from build123d import *

# Parameters (mm, degrees)
SKETCH_1_W           = 300
SKETCH_1_H           = 100
EXTRUDE_1_DEPTH      = 16
SKETCH_2_W           = 30
SKETCH_2_H           = 30
CUT_EXTRUDE_1_DEPTH  = 8
SKETCH_3_R           = 12.5
CUT_EXTRUDE_2_DEPTH  = 14
CUT_EXTRUDE_3_REACH  = 318.632
SKETCH_4_W           = 50
SKETCH_4_H           = 35
SKETCH_7_W           = 35
SKETCH_7_H           = 16
EXTRUDE_2_DEPTH      = 20
SKETCH_8_W           = 35
SKETCH_8_H           = 16
EXTRUDE_3_DEPTH      = 20
SKETCH_9_W           = 20
SKETCH_9_H           = 10
EXTRUDE_4_DEPTH      = 25
FILLET_1_R           = 1
FILLET_2_R           = 1
SKETCH_13_W          = 35
SKETCH_13_H          = 16
EXTRUDE_6_DEPTH      = 4
SKETCH_14_W          = 35
SKETCH_14_H          = 16
EXTRUDE_7_DEPTH      = 4
SKETCH_17_W          = 35
SKETCH_17_H          = 16
EXTRUDE_8_DEPTH      = 1
SKETCH_18_W          = 35
SKETCH_18_H          = 16
EXTRUDE_9_DEPTH      = 1
SKETCH_19_R          = 2.25
CUT_EXTRUDE_8_DEPTH  = 5
CUT_EXTRUDE_START    = -5
SKETCH_20_R          = 2.25
CUT_EXTRUDE_9_DEPTH  = 5
SKETCH_21_R          = 1.45
CUT_EXTRUDE_10_DEPTH = 5
SKETCH_22_R          = 2.25
CUT_EXTRUDE_11_DEPTH = 5
SKETCH_23_R          = 1.45
CUT_EXTRUDE_12_DEPTH = 5
SKETCH_24_R          = 2.25
CUT_EXTRUDE_13_DEPTH = 5


with BuildPart() as part:
    # 草图1 → 凸台-拉伸1 (new body)
    with BuildSketch(Plane(origin=(0, 0, 0), x_dir=(1, 0, 0), z_dir=(0, 1, 0))):
        with Locations((-150, 50)):
            Rectangle(SKETCH_1_W, SKETCH_1_H)
    extrude(amount=EXTRUDE_1_DEPTH)

    # 草图2 → 切除-拉伸1 (cut)
    with BuildSketch(Plane(origin=(0, 16, 0), x_dir=(1, 0, 0), z_dir=(0, 1, 0))):
        with Locations((-150, 50)):
            Rectangle(SKETCH_2_W, SKETCH_2_H)
    extrude(amount=-CUT_EXTRUDE_1_DEPTH, mode=Mode.SUBTRACT)

    # 草图3 → 切除-拉伸2 (cut)
    with BuildSketch(Plane(origin=(0, 8, 0), x_dir=(1, 0, 0), z_dir=(0, 1, 0))):
        with Locations(Location((-150, 50, 0), (0, 0, 270))):
            Circle(SKETCH_3_R)
    extrude(amount=-CUT_EXTRUDE_2_DEPTH, mode=Mode.SUBTRACT)

    # 草图4 → 切除-拉伸3 (cut, up to next)
    with BuildSketch(Plane(origin=(0, 16, 0), x_dir=(1, 0, 0), z_dir=(0, 1, 0)), mode=Mode.PRIVATE) as cut_extrude_3_sk1:
        with Locations((-270, 72.5)):
            Rectangle(SKETCH_4_W, SKETCH_4_H)
    cut_extrude_3_tool1 = extrude(cut_extrude_3_sk1.sketch, amount=-CUT_EXTRUDE_3_REACH, mode=Mode.PRIVATE) & part.part
    # 草图4 → 切除-拉伸3 (cut, up to next)
    with BuildSketch(Plane(origin=(0, 16, 0), x_dir=(1, 0, 0), z_dir=(0, 1, 0)), mode=Mode.PRIVATE) as cut_extrude_3_sk2:
        with Locations((-270, 27.5)):
            Rectangle(SKETCH_4_W, SKETCH_4_H)
    cut_extrude_3_tool2 = extrude(cut_extrude_3_sk2.sketch, amount=-CUT_EXTRUDE_3_REACH, mode=Mode.PRIVATE) & part.part
    # 草图4 → 切除-拉伸3 (cut, up to next)
    with BuildSketch(Plane(origin=(0, 16, 0), x_dir=(1, 0, 0), z_dir=(0, 1, 0)), mode=Mode.PRIVATE) as cut_extrude_3_sk3:
        with Locations((-210, 72.5)):
            Rectangle(SKETCH_4_W, SKETCH_4_H)
    cut_extrude_3_tool3 = extrude(cut_extrude_3_sk3.sketch, amount=-CUT_EXTRUDE_3_REACH, mode=Mode.PRIVATE) & part.part
    # 草图4 → 切除-拉伸3 (cut, up to next)
    with BuildSketch(Plane(origin=(0, 16, 0), x_dir=(1, 0, 0), z_dir=(0, 1, 0)), mode=Mode.PRIVATE) as cut_extrude_3_sk4:
        with Locations((-210, 27.5)):
            Rectangle(SKETCH_4_W, SKETCH_4_H)
    cut_extrude_3_tool4 = extrude(cut_extrude_3_sk4.sketch, amount=-CUT_EXTRUDE_3_REACH, mode=Mode.PRIVATE) & part.part
    # 草图4 → 切除-拉伸3 (cut, up to next)
    with BuildSketch(Plane(origin=(0, 16, 0), x_dir=(1, 0, 0), z_dir=(0, 1, 0)), mode=Mode.PRIVATE) as cut_extrude_3_sk5:
        with Locations((-30, 27.5)):
            Rectangle(SKETCH_4_W, SKETCH_4_H)
    cut_extrude_3_tool5 = extrude(cut_extrude_3_sk5.sketch, amount=-CUT_EXTRUDE_3_REACH, mode=Mode.PRIVATE) & part.part
    # 草图4 → 切除-拉伸3 (cut, up to next)
    with BuildSketch(Plane(origin=(0, 16, 0), x_dir=(1, 0, 0), z_dir=(0, 1, 0)), mode=Mode.PRIVATE) as cut_extrude_3_sk6:
        with Locations((-90, 27.5)):
            Rectangle(SKETCH_4_W, SKETCH_4_H)
    cut_extrude_3_tool6 = extrude(cut_extrude_3_sk6.sketch, amount=-CUT_EXTRUDE_3_REACH, mode=Mode.PRIVATE) & part.part
    # 草图4 → 切除-拉伸3 (cut, up to next)
    with BuildSketch(Plane(origin=(0, 16, 0), x_dir=(1, 0, 0), z_dir=(0, 1, 0)), mode=Mode.PRIVATE) as cut_extrude_3_sk7:
        with Locations((-90, 72.5)):
            Rectangle(SKETCH_4_W, SKETCH_4_H)
    cut_extrude_3_tool7 = extrude(cut_extrude_3_sk7.sketch, amount=-CUT_EXTRUDE_3_REACH, mode=Mode.PRIVATE) & part.part
    # 草图4 → 切除-拉伸3 (cut, up to next)
    with BuildSketch(Plane(origin=(0, 16, 0), x_dir=(1, 0, 0), z_dir=(0, 1, 0)), mode=Mode.PRIVATE) as cut_extrude_3_sk8:
        with Locations((-30, 72.5)):
            Rectangle(SKETCH_4_W, SKETCH_4_H)
    cut_extrude_3_tool8 = extrude(cut_extrude_3_sk8.sketch, amount=-CUT_EXTRUDE_3_REACH, mode=Mode.PRIVATE) & part.part
    add(cut_extrude_3_tool1.solids().sort_by_distance((-270, 16, -72.5))[0], mode=Mode.SUBTRACT)
    add(cut_extrude_3_tool2.solids().sort_by_distance((-270, 16, -27.5))[0], mode=Mode.SUBTRACT)
    add(cut_extrude_3_tool3.solids().sort_by_distance((-210, 16, -72.5))[0], mode=Mode.SUBTRACT)
    add(cut_extrude_3_tool4.solids().sort_by_distance((-210, 16, -27.5))[0], mode=Mode.SUBTRACT)
    add(cut_extrude_3_tool5.solids().sort_by_distance((-30, 16, -27.5))[0], mode=Mode.SUBTRACT)
    add(cut_extrude_3_tool6.solids().sort_by_distance((-90, 16, -27.5))[0], mode=Mode.SUBTRACT)
    add(cut_extrude_3_tool7.solids().sort_by_distance((-90, 16, -72.5))[0], mode=Mode.SUBTRACT)
    add(cut_extrude_3_tool8.solids().sort_by_distance((-30, 16, -72.5))[0], mode=Mode.SUBTRACT)

    # 草图7 → 凸台-拉伸2 (add)
    with BuildSketch(Plane.ZY.offset(185)):
        with Locations((-27.5, 8)):
            Rectangle(SKETCH_7_W, SKETCH_7_H)
        with Locations((-72.5, 8)):
            Rectangle(SKETCH_7_W, SKETCH_7_H)
    extrude(amount=EXTRUDE_2_DEPTH)

    # 草图8 → 凸台-拉伸3 (add)
    with BuildSketch(Plane(origin=(-115, 0, 0), x_dir=(0, 0, -1), z_dir=(1, 0, 0))):
        with Locations((27.5, 8)):
            Rectangle(SKETCH_8_W, SKETCH_8_H)
        with Locations((72.5, 8)):
            Rectangle(SKETCH_8_W, SKETCH_8_H)
    extrude(amount=EXTRUDE_3_DEPTH)

    # 草图9 → 凸台-拉伸4 (add)
    with BuildSketch(Plane.XZ):
        with Locations((-250, -95)):
            Rectangle(SKETCH_9_W, SKETCH_9_H)
    extrude(amount=EXTRUDE_4_DEPTH)

    # 圆角1
    fillet_1_edges = [part.edges().sort_by_distance(p)[0] for p in [
        (-150, 8, -62.5),
    ]]
    fillet(fillet_1_edges, radius=FILLET_1_R)

    # 圆角2
    fillet_2_edges = [part.edges().sort_by_distance(p)[0] for p in [
        (-135, 16, -50),
        (-150, 16, -65),
        (-165, 16, -50),
        (-150, 16, -35),
    ]]
    fillet(fillet_2_edges, radius=FILLET_2_R)

    # 草图13 → 凸台-拉伸6 (add)
    with BuildSketch(Plane.ZY.offset(5)):
        with Locations((-72.5, 8)):
            Rectangle(SKETCH_13_W, SKETCH_13_H)
        with Locations((-27.5, 8)):
            Rectangle(SKETCH_13_W, SKETCH_13_H)
    extrude(amount=EXTRUDE_6_DEPTH)

    # 草图14 → 凸台-拉伸7 (add)
    with BuildSketch(Plane(origin=(-295, 0, 0), x_dir=(0, 0, -1), z_dir=(1, 0, 0))):
        with Locations((72.5, 8)):
            Rectangle(SKETCH_14_W, SKETCH_14_H)
        with Locations((27.5, 8)):
            Rectangle(SKETCH_14_W, SKETCH_14_H)
    extrude(amount=EXTRUDE_7_DEPTH)

    # 草图17 → 凸台-拉伸8 (add)
    with BuildSketch(Plane(origin=(-291, 0, 0), x_dir=(0, 0, -1), z_dir=(1, 0, 0))):
        with Locations((27.5, 8)):
            Rectangle(SKETCH_17_W, SKETCH_17_H)
        with Locations((72.5, 8)):
            Rectangle(SKETCH_17_W, SKETCH_17_H)
    extrude(amount=EXTRUDE_8_DEPTH)

    # 草图18 → 凸台-拉伸9 (add)
    with BuildSketch(Plane.ZY.offset(9)):
        with Locations((-27.5, 8)):
            Rectangle(SKETCH_18_W, SKETCH_18_H)
        with Locations((-72.5, 8)):
            Rectangle(SKETCH_18_W, SKETCH_18_H)
    extrude(amount=EXTRUDE_9_DEPTH)

    # 草图19 → 切除-拉伸8 (cut)
    with BuildSketch(Plane(origin=(0, 16, 0), x_dir=(1, 0, 0), z_dir=(0, 1, 0))):
        with Locations(Location((-295, 95, 0), (0, 0, 270))):
            Circle(SKETCH_19_R)
        with Locations(Location((-295, 5, 0), (0, 0, 90))):
            Circle(SKETCH_19_R)
        with Locations(Location((-5, 5, 0), (0, 0, 270))):
            Circle(SKETCH_19_R)
        with Locations(Location((-5, 95, 0), (0, 0, 90))):
            Circle(SKETCH_19_R)
    extrude(amount=-CUT_EXTRUDE_8_DEPTH, mode=Mode.SUBTRACT)

    # 草图20 → 切除-拉伸9 (cut)
    with BuildSketch(Plane.XZ.offset(CUT_EXTRUDE_START)):
        with Locations(Location((-295, -95, 0), (0, 0, 90))):
            Circle(SKETCH_20_R)
        with Locations(Location((-295, -5, 0), (0, 0, 270))):
            Circle(SKETCH_20_R)
        with Locations(Location((-5, -95, 0), (0, 0, 270))):
            Circle(SKETCH_20_R)
        with Locations(Location((-5, -5, 0), (0, 0, 90))):
            Circle(SKETCH_20_R)
    extrude(amount=CUT_EXTRUDE_9_DEPTH, mode=Mode.SUBTRACT)

    # 草图21 → 切除-拉伸10 (cut)
    with BuildSketch(Plane(origin=(-100.276222054, 16, -200.091791604), x_dir=(-0.00184091553368713, 0, -0.9999983055135633), z_dir=(0, 1, 0))):
        with Locations(Location((-104.543338614, 26.416278164, 0), (0, 0, 179.89452325))):
            Circle(SKETCH_21_R)
        with Locations(Location((-121.543309808, 26.447573728, 0), (0, 0, 179.89452325))):
            Circle(SKETCH_21_R)
        with Locations(Location((-121.456786778, 73.447494087, 0), (0, 0, 179.89452325))):
            Circle(SKETCH_21_R)
        with Locations(Location((-104.456815584, 73.416198523, 0), (0, 0, 179.89452325))):
            Circle(SKETCH_21_R)
    extrude(amount=-CUT_EXTRUDE_10_DEPTH, mode=Mode.SUBTRACT)

    # 草图22 → 切除-拉伸11 (cut)
    with BuildSketch(Plane(origin=(0, 16, 0), x_dir=(1, 0, 0), z_dir=(0, 1, 0))):
        with Locations(Location((-173.5, 95.5, 0), (0, 0, 270))):
            Circle(SKETCH_22_R)
        with Locations(Location((-173.5, 78.5, 0), (0, 0, 270))):
            Circle(SKETCH_22_R)
        with Locations(Location((-126.5, 95.5, 0), (0, 0, 270))):
            Circle(SKETCH_22_R)
        with Locations(Location((-126.5, 78.5, 0), (0, 0, 270))):
            Circle(SKETCH_22_R)
    extrude(amount=-CUT_EXTRUDE_11_DEPTH, mode=Mode.SUBTRACT)

    # 草图23 → 切除-拉伸12 (cut)
    with BuildSketch(Plane(origin=(-100.276222054, 16, -200.091791604), x_dir=(-0.00184091553368713, 0, -0.9999983055135633), z_dir=(0, 1, 0))):
        with Locations(Location((-119.069051565, 12.462168574, 0), (0, 0, 179.89452325))):
            Circle(SKETCH_23_R)
        with Locations(Location((-145.069007508, 12.510032378, 0), (0, 0, 179.89452325))):
            Circle(SKETCH_23_R)
        with Locations(Location((-144.931009437, 87.471558467, 0), (0, 0, 179.89452325))):
            Circle(SKETCH_23_R)
        with Locations(Location((-118.931053493, 87.423694663, 0), (0, 0, 179.89452325))):
            Circle(SKETCH_23_R)
    extrude(amount=-CUT_EXTRUDE_12_DEPTH, mode=Mode.SUBTRACT)

    # 草图24 → 切除-拉伸13 (cut)
    with BuildSketch(Plane(origin=(0, 16, 0), x_dir=(1, 0, 0), z_dir=(0, 1, 0))):
        with Locations(Location((-187.480826555, 81, 0), (0, 0, 270))):
            Circle(SKETCH_24_R)
        with Locations(Location((-187.480826555, 55, 0), (0, 0, 270))):
            Circle(SKETCH_24_R)
        with Locations(Location((-112.519173445, 81, 0), (0, 0, 270))):
            Circle(SKETCH_24_R)
        with Locations(Location((-112.519173445, 55, 0), (0, 0, 270))):
            Circle(SKETCH_24_R)
    extrude(amount=-CUT_EXTRUDE_13_DEPTH, mode=Mode.SUBTRACT)


solid = part.part
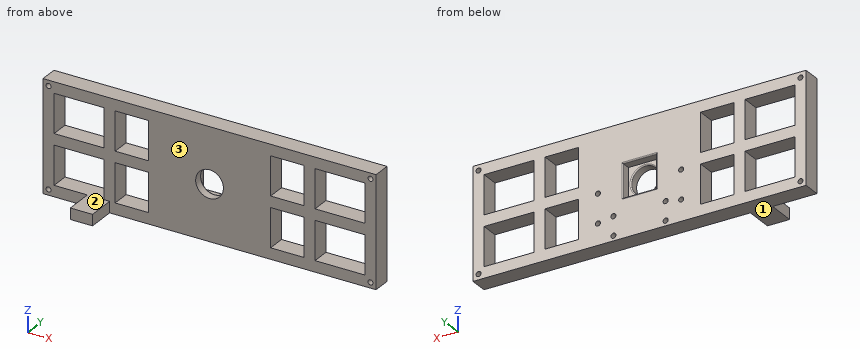
Input: part model. Units: mm. Frame: model coordinates. Face numbers are marked on the shaded views. Give positions to 0.01 mm unless a question says otherwise; leave off trailing zeros. Order: outer loops, then holes, each group sorted by start corner. A loop starts at its lowest first (then second) coordinate and runs counter-clockwise, first axis right, second up. Notation, with made-up numbers: M 84,15.25 L 119,15.25 A13 cw 119,35.25 Z; hole C -24.75,86.25 d8. An arc over 180 degrees is marked long. Answer as a JSON object with one key per item and string values.
1. Cut plane A-A, the plane x = -50. Output: boundary loops of the cut face in (y, z).
Result sheet:
{"outline": "M 0,-100 L 16,-100 L 16,-90 L 0,-90 Z; M 0,-55 L 16,-55 L 16,-45 L 0,-45 Z; M 0,-10 L 16,-10 L 16,0 L 0,0 Z"}
2. Cut plane B-B, the plane y = -9. Output: boundary loops of the cut face in (x, z).
Result sheet:
{"outline": "M -260,-100 L -240,-100 L -240,-90 L -260,-90 Z"}
3. Pull-direction query (Z, two-part tool) for the marked faces 1, 2 and 3; classes: +Z half, -Z half, draft (parallel to the pull), parting line (faces both ways), or undercut.
Result sheet:
{"face 1": "-Z half", "face 2": "undercut", "face 3": "draft"}
4. Ray query, line 1 (Z direction, x = -31.5, y = 2.5); line 2 (Z direction, x = -295, y = 3); line 3 (X direction, y = 13.4, z = -95.5). Return the intervals inside material, ascending. Write a range as [from, to].
Result sheet:
{"line 1": "[-100, -90], [-55, -45], [-10, 0]", "line 2": "[-100, -97.25], [-92.75, -7.25], [-2.75, 0]", "line 3": "[-300, -297.19], [-292.81, -175.75], [-171.25, -128.75], [-124.25, -7.19], [-2.81, 0]"}
5. First-contact query: P1, Ø1.3, axis at x = -5, z = -5.5, coming from the +Y side; P2, Ø3.5, axis at x = -294, z = -96, coming from the -Y side; P3, Ø6, axis at y = -3.5, z = -30.5, coming from the -X side. Flat tips, straight axial feed; report the tip coordinate or a pass-through.
Result sheet:
{"P1": "y = 11", "P2": "y = 0", "P3": "through"}
6. Cut plane C-C, the plane x = -102. Output: boundary loops of the cut face in (y, z).
Result sheet:
{"outline": "M 0,-100 L 16,-100 L 16,0 L 0,0 Z"}
